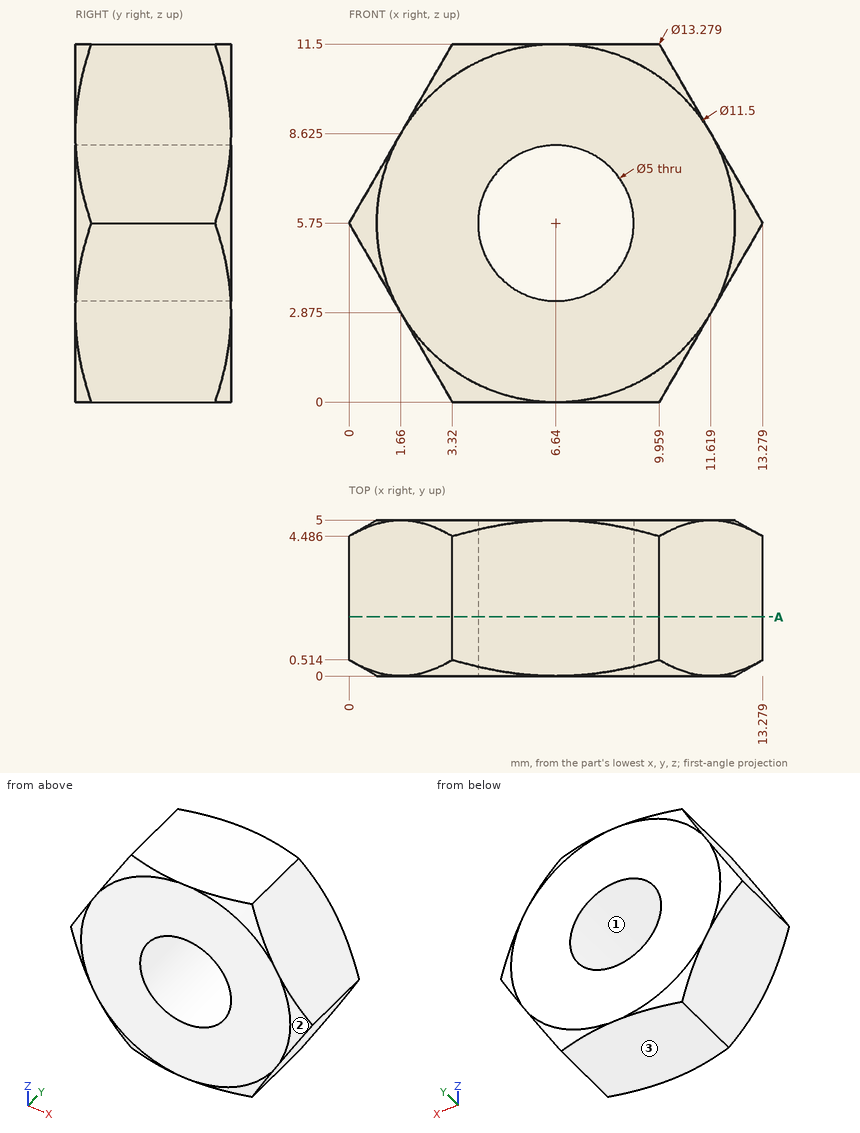
Part print with two shaded views. Sizes in mm from the minimum x, y, z corner. Round coordinates to 2 decimals unless told otherwise and drop trailing zeros. Order: outer loops, then holes, each group sorted by start corner. A loop starts at its lowest first (then second) coordinate and runs counter-clockwise, first axis right, second up. Notation, with made-up numbers: M 64.5,66 L 72.5,66 A31 cw 72.5,96 Z; hole C 37,28.25 d3. An arc over 180 degrees is marked long. Use CSV: the item, a comma, the result in double quotes.
Item 1: Probe probe 1 along Z at (x, y) = (8.25, 0.75); probe 2 along X at (y, z) = (3.8, 7) (1 decimal); probe 3 along X at (y, z) = (2.5, 6) (1 decimal). List the from-to ranges inside material, lowest first.
Worked answers:
probe 1,"0 to 3.84, 7.66 to 11.5"
probe 2,"0.7 to 4.5, 8.8 to 12.6"
probe 3,"0.1 to 4.2, 9.1 to 13.1"
Item 2: Pin check, flat tip, straight feed: pin 1 (3 mm diameter, centred on y = 2, z = 5.5, fed in from -X). Stop position of the tip, or through.
Worked answers:
pin 1,"x = 0"
Item 3: Pull direction Z, two halves, no side cores. Call the marked faces 1, 2 and 3: released by +Z, released by -Z, zero draft, split by the parting line, or undercut.
Worked answers:
face 1,"undercut"
face 2,"split by the parting line"
face 3,"released by -Z"
Item 4: Saw through at A-A (y = 1.9). List the corners of the cut face in (x, z).
Worked answers:
outline,"M 0,5.75 L 3.32,0 L 9.96,0 L 13.28,5.75 L 9.96,11.5 L 3.32,11.5 Z; hole C 6.64,5.75 d5"
